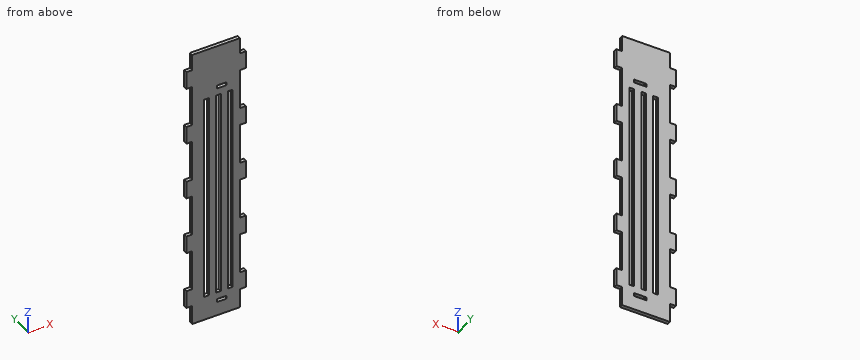
Autodesk Inventor part; units mm, degrees
ref_plane "YZ Plane" through (0, 0, 0) normal (1, 0, 0) x (0, 1, 0)
ref_plane "XZ Plane" through (0, 0, 0) normal (0, 1, 0) x (-1, 0, 0)
ref_plane "XY Plane" through (0, 0, 0) normal (0, 0, 1) x (1, 0, 0)
sketch "Sketch1" plane through (0, 0, 0) normal (0, 1, 0) x (-1, 0, 0)
  line L0 (20.15, 134.75) -> (-20.15, 134.75)
  line L1 (-20.15, 134.75) -> (-20.15, -110.95)
  line L2 (-20.15, -110.95) -> (20.15, -110.95)
  line L3 (20.15, -110.95) -> (20.15, 134.75)
  line L4 (20.15, 0) -> (-20.15, 0) construction
  line L5 (0, -110.95) -> (0, 134.75) construction
  point P0 (0, 0)
  point P1 (0, 0)
  dimension "d57" = 40.3
  dimension "d58" = 110.95
  dimension "d59" = 134.75
extrude "Extrusion1" add sketch "Sketch1" along normal blind 3
sketch "Sketch3" plane through (0, 0, 0) normal (0, -1, 0) x (1, 0, 0)
  line L0 (20.15, -110.95) -> (-20.15, -110.95)
  line L1 (20.15, 134.75) -> (20.15, -110.95)
  line L2 (-20.15, -110.95) -> (-20.15, 134.75)
  line L3 (-25.15, -79.15) -> (-20.15, -79.15)
  line L4 (-20.15, -79.15) -> (-20.15, -94.45)
  line L5 (-20.15, -94.45) -> (-25.15, -94.45)
  line L6 (-25.15, -94.45) -> (-25.15, -79.15)
  line L7 (-25.15, -79.15) -> (-20.15, -94.45) construction
  line L8 (-20.15, -79.15) -> (-25.15, -94.45) construction
  line L9 (25.15, -94.45) -> (20.15, -94.45)
  line L10 (20.15, -94.45) -> (20.15, -79.15)
  line L11 (20.15, -79.15) -> (25.15, -79.15)
  line L12 (25.15, -79.15) -> (25.15, -94.45)
  line L13 (25.15, -94.45) -> (20.15, -79.15) construction
  line L14 (20.15, -94.45) -> (25.15, -79.15) construction
  point P0 (0, 0)
  point P1 (-22.65, -86.8)
  point P2 (22.65, -86.8)
  point P3 (20.15, -86.8)
  dimension "d61" = 15.3
  dimension "d64" = 5
  dimension "d65" = 15.3
  dimension "d78" = 24.15
  dimension "d79" = 24.15
  dimension "d97" = 5
extrude "Extrusion3" add sketch "Sketch3" against normal blind 3
pattern_linear "Rectangular Pattern1" count 5 spacing 50 along (0, 0, 1) of "Extrusion3"
sketch "Sketch4" plane through (0, 0, 0) normal (0, -1, 0) x (1, 0, 0)
  line L0 (20.15, -110.95) -> (-20.15, -110.95)
  line L1 (1, -96.15) -> (9, -96.15)
  line L2 (9, -96.15) -> (9, -98.85)
  line L3 (9, -98.85) -> (1, -98.85)
  line L4 (1, -98.85) -> (1, -96.15)
  line L5 (1, -96.15) -> (9, -98.85) construction
  line L6 (9, -96.15) -> (1, -98.85) construction
  line L7 (5, -118.696) -> (5, 153.6812) construction
  point P0 (5, -97.5)
  point P1 (5, -97.5)
  point P2 (5, -97.5)
  point P3 (5, -97.5)
  point P4 (0, 0)
  dimension "d69" = 8
  dimension "d70" = 2.7
  dimension "d98" = 13.45
  dimension "d100" = 5
extrude "Extrusion4" cut sketch "Sketch4" against normal blind 3
pattern_linear "Rectangular Pattern2" count 2 spacing 195 along (0, 0, 1) of "Extrusion4"
sketch "Sketch8" plane through (0, 3, 0) normal (0, 1, 0) x (1, 0, 0)
  line L0 (-10, -90) -> (-6, -90)
  line L1 (-6, -90) -> (-6, 90)
  line L2 (-6, 90) -> (-10, 90)
  line L3 (-10, 90) -> (-10, -90)
  line L4 (-10, -90) -> (-6, 90) construction
  line L5 (-6, -90) -> (-10, 90) construction
  point P0 (0, 0)
  point P1 (-8, 0)
  dimension "d82" = 4
  dimension "d83" = 180
  dimension "d84" = 6
extrude "Extrusion5" cut sketch "Sketch8" against normal through all
sketch "Sketch9" plane through (0, 3, 0) normal (0, 1, 0) x (1, 0, 0)
  line L0 (1, 96.15) -> (1, 98.85)
  line L1 (1, 98.85) -> (9, 98.85)
  line L2 (9, 98.85) -> (9, 96.15)
  line L3 (9, 96.15) -> (1, 96.15)
  line L4 (-0.35, 96.15) -> (10.35, 96.15)
  line L5 (10.35, 96.15) -> (10.35, 98.85)
  line L6 (10.35, 98.85) -> (-0.35, 98.85)
  line L7 (-0.35, 98.85) -> (-0.35, 96.15)
  line L8 (-0.35, 96.15) -> (10.35, 98.85) construction
  line L9 (10.35, 96.15) -> (-0.35, 98.85) construction
  line L10 (1, 98.85) -> (9, 96.15) construction
  line L11 (9, 96.15) -> (9, 98.85) construction
  line L12 (9, 98.85) -> (1, 96.15) construction
  point P0 (0, 0)
  point P1 (5, 97.5)
  point P2 (5, 97.5)
  dimension "d90" = 10.7
  dimension "d91" = 2.7
extrude "Extrusion6" cut sketch "Sketch9" against normal blind 1.5 contours L4 L7 L6 L0 | L2 L6 L5 L4
pattern_linear "Rectangular Pattern4" count 2 spacing 195 along (0, 0, 1) of "Extrusion6"
pattern_linear "Rectangular Pattern5" count 3 spacing 10 along (1, 0, 0) of "Extrusion5"
equation "\"kerf\" = 0.15"
properties part number "Panel3" material "Acrylic, Clear"
Geometry: final body of the model. Coordinates: model frame, mm. Round coordinates to 2 decimals unless told otherwise and drop trailing zeros. Loops run counter-clockwise (first coordinate to the right, second up) from the corner with the lowest first, then second, coordinate; pieces in that order, holes last. Notation, with made-up numbers: M 11.25,57 L 21.25,57 A13 cw 21.25,68 Z; hole C -4.75,27.25 d3. An arc over 180 degrees is marked long. Put each result on its own line as item: value. Start each with the question number.
(1) Contact query for flat-ended pins moving along their axis: pin 1 Ø0.7 at (x, z) = (0.5, 97) entering from +Y; pin 2 Ø1.5 at (x, y) = (22.5, 2) entering from +Z; pin 3 Ø1 at (y, z) = (2, -16) entering from +X. Output: stop coordinate, or through.
(2) Section query B-B (y = 1). State how many separate pieces and enclosed holes the cut face has, then the cut area to 3 significant figures.
(3) Material intervals for line 1 along X through (y, z) = (1.4, 68.5); line 2 along X through (y, z) = (1.8, -12); line 3 along Z through (x, y) = (8, 1.65), sorted ascending. Write a range as [from, to].
(4) Section query A-A (z = 73). Return loops of the section in (x, y), then the cut area to 3 significant figures.
Findings below:
1. pin 1: stops at y = 1.5
1. pin 2: stops at z = 120.85
1. pin 3: stops at x = 20.15
2. separate pieces: 1
2. enclosed holes: 5
2. area: 8,460 mm2
3. line 1: x = [-25.15, -10], [-6, 0], [4, 10], [14, 25.15]
3. line 2: x = [-20.15, -10], [-6, 0], [4, 10], [14, 20.15]
3. line 3: z = [-110.95, -98.85], [-96.15, 96.15], [98.85, 134.75]
4. outline: M -20.15,0 L -10,0 L -10,3 L -20.15,3 Z; M -6,0 L 0,0 L 0,3 L -6,3 Z; M 4,0 L 10,0 L 10,3 L 4,3 Z; M 14,0 L 20.15,0 L 20.15,3 L 14,3 Z
4. area: 84.9 mm2
